from build123d import *

# Parameters (mm, degrees)
EXTRUDE_1_DEPTH             = 948
SKETCH_2_W                  = 200
SKETCH_2_H                  = 325
EXTRUDE_2_DEPTH             = 20
SKETCH_3_W                  = 200
SKETCH_3_H                  = 325
EXTRUDE_3_DEPTH             = 20
SKETCH_4_R                  = 11.5
CUT_EXTRUDE_1_DEPTH         = 1027.912970996
PATTERN_LINEAR_1_COUNT      = 2
PATTERN_LINEAR_1_PITCH      = 125
PATTERN_LINEAR_1_COUNT_DIR2 = 3
PATTERN_LINEAR_1_PITCH_DIR2 = 125


with BuildPart() as part:
    # 草图1 → 凸台-拉伸1 (new body)
    with BuildSketch(Plane.XY):
        Polygon((0, 120), (0, 110), (65, 110), (65, 10), (0, 10), (0, 0), (140, 0), (140, 10), (75, 10), (75, 110), (140, 110), (140, 120), align=None)
    extrude(amount=EXTRUDE_1_DEPTH)

    # 草图2 → 凸台-拉伸2 (add)
    with BuildSketch(Plane.XY.offset(948)):
        with Locations((70, 60)):
            Rectangle(SKETCH_2_W, SKETCH_2_H)
    extrude(amount=EXTRUDE_2_DEPTH)

    # 草图3 → 凸台-拉伸3 (add)
    with BuildSketch(Plane(origin=(0, 0, 0), x_dir=(-1, 0, 0), z_dir=(0, 0, -1))):
        with Locations((-70, 60)):
            Rectangle(SKETCH_3_W, SKETCH_3_H)
    extrude(amount=EXTRUDE_3_DEPTH)

    # 草图4 → 切除-拉伸1 (cut, through all)
    with BuildSketch(Plane.XY.offset(968)):
        with Locations((7.5, 185)):
            Circle(SKETCH_4_R)
    cut_extrude_1 = extrude(amount=-CUT_EXTRUDE_1_DEPTH, mode=Mode.SUBTRACT)

    # 阵列(线性)1: Cut-Extrude 1 2 × 3
    with Locations(*[(i * PATTERN_LINEAR_1_PITCH, -j * PATTERN_LINEAR_1_PITCH_DIR2, 0) for i in range(PATTERN_LINEAR_1_COUNT) for j in range(PATTERN_LINEAR_1_COUNT_DIR2) if (i, j) != (0, 0)]):
        add(cut_extrude_1, mode=Mode.SUBTRACT)


solid = part.part
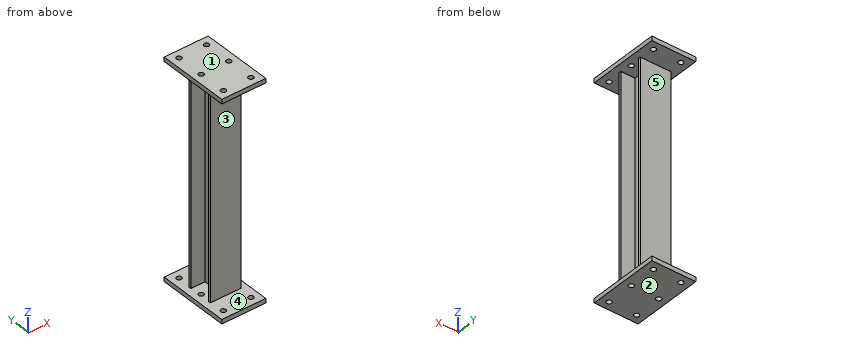
Geometry: final body of the model. Coordinates: model frame, mm. Face numbers are marked on the shaded views. A direction names the side the tool comes from. Give positions to 0.01 mm unless a question says otherwise; leave off trailing zeros. Write each loop counter-clockwise with the first axis right and the second up, starting at its lowest first coordinate (ties: lowest second). Pieces come first, ordered by that corner, then holes.
(1) Cut plane A-A, the plane y = -65. Return loops of the section in (x, z).
(2) Access query for the marked faces 4 and 5. Directions: +Z, -Z, +X, -X, +Y, -Y. A direction counts if a zero-diameter tool reaches every point of the face in a straight line with its end or side. Return the directions, or none.
(3) Cut plane C-C, the plane x = 111.5. Return loops of the section in (y, z).
(4) First-contact query: P1, Ø6, axis at x = 75, z = 442.5, coming from the +Y side; P2, Ø1.5, axis at y = 27, z = 467.5, coming from the +X side; P3, Ø8, axis at y = 116.5, z = 652.5, coming from the -X side. Flat tips, straight axial feed; report the tip coordinate or a pass-through.
(5) Cut plane B-B, the plane y = 154. Return loops of the section in (x, z).
(6) Mould query, pull axis Z, two halves, no side actions, for the marked faces 1, 2 and 3. Classes: released by +Z, released by -Z, zero draft, split by the parting line, or undercut.
(7) Cut plane D-D, the plane z = 416.5. Return loops of the section in (x, y), then the cut area to 3 significant figures.
(8) Ray query, line 1 (Y direction, x = 132.5, z = -6.25); line 2 (Z direction, x = -8, y = -65); line 3 (Y direction, x = 97.5, z = 139). Return the intervals inside material, ascending.
Values follow:
1. outline: (-30, -20) - (-4, -20) - (-4, 0) - (-30, 0) - close; (-30, 948) - (-4, 948) - (-4, 968) - (-30, 968) - close; (19, -20) - (121, -20) - (121, 0) - (19, 0) - close; (19, 948) - (121, 948) - (121, 968) - (19, 968) - close; (144, -20) - (170, -20) - (170, 0) - (144, 0) - close; (144, 948) - (170, 948) - (170, 968) - (144, 968) - close
2. face 4: none
2. face 5: +X, -X, +Y
3. outline: (-102.5, -20) - (222.5, -20) - (222.5, 0) - (120, 0) - (120, 948) - (222.5, 948) - (222.5, 968) - (-102.5, 968) - (-102.5, 948) - (0, 948) - (0, 0) - (-102.5, 0) - close; hole (10, 0) - (110, 0) - (110, 948) - (10, 948) - close
4. P1: stops at y = 120
4. P2: stops at x = 75
4. P3: stops at x = 0
5. outline: (-30, -20) - (170, -20) - (170, 0) - (-30, 0) - close; (-30, 948) - (170, 948) - (170, 968) - (-30, 968) - close
6. face 1: released by +Z
6. face 2: released by -Z
6. face 3: undercut
7. outline: (0, 0) - (140, 0) - (140, 10) - (75, 10) - (75, 110) - (140, 110) - (140, 120) - (0, 120) - (0, 110) - (65, 110) - (65, 10) - (0, 10) - close
7. area: 3,800 mm2
8. line 1: y = -102.5 to -76.5, -53.5 to 48.5, 71.5 to 173.5, 196.5 to 222.5
8. line 2: z = -20 to 0, 948 to 968
8. line 3: y = 0 to 10, 110 to 120
